```python
from build123d import *

# Parameters (mm, degrees)
SKETCH_W        = 74.53746
SKETCH_H        = 38
PAD_DEPTH       = 2
SKETCH001_W     = 6.85
SKETCH001_H     = 15
PAD001_DEPTH    = 20
SKETCH002_R     = 1.5
POCKET_DEPTH    = 17
SKETCH003_R     = 1.5
PAD002_DEPTH    = 2
SKETCH004_R     = 2.95
PAD003_DEPTH    = 5
SKETCH005_R     = 2.7
SKETCH005_R_2   = 1.5
PAD004_DEPTH    = 2
SKETCH006_W     = 7.7
SKETCH006_H     = 20
SKETCH006_R     = 2.7
PAD005_DEPTH    = 3
SKETCH007_R     = 1.5
PAD006_DEPTH    = 13
SKETCH008_R     = 1.5
PAD007_DEPTH    = 13
FILLET_R        = 3
FILLET001_R     = 5
FILLET002_R     = 1
CHAMFER_SIZE    = 2
CHAMFER001_SIZE = 2


with BuildPart() as body:
    # Sketch → Pad (new body)
    with BuildSketch(Plane.XY):
        Rectangle(SKETCH_W, SKETCH_H)
    extrude(amount=PAD_DEPTH)

    # Sketch001 (on Face6 of Pad) → Pad001 (join)
    with BuildSketch(Plane.XY.offset(2)):
        with Locations((33.84373, -1.3)):
            Rectangle(SKETCH001_W, SKETCH001_H)
        with Locations((-13.60627, -1.3)):
            Rectangle(SKETCH001_W, SKETCH001_H)
    extrude(amount=PAD001_DEPTH)

    # Sketch002 (on Face12 of Pad001) → Pocket (cut)
    with BuildSketch(Plane.XZ.offset(8.8)):
        with Locations((-14.03127, 17)):
            Circle(SKETCH002_R)
        with Locations((-14.03127, 7)):
            Circle(SKETCH002_R)
        with Locations((34.26873, 17)):
            Circle(SKETCH002_R)
        with Locations((34.26873, 7)):
            Circle(SKETCH002_R)
    extrude(amount=-POCKET_DEPTH, mode=Mode.SUBTRACT)

    # Sketch003 (on Face6 of Pocket) → Pad002 (join)
    with BuildSketch(Plane.XZ.offset(19)):
        with BuildLine():
            Line((37.26873, 0), (-37.26873, 0))
            ThreePointArc((-37.26873, 22), (-48.26873, 11), (-37.26873, 0))
            Line((-37.26873, 22), (27.26873, 22))
            ThreePointArc((37.26873, 12), (34.339798, 19.071068), (27.26873, 22))
            Line((37.26873, 12), (37.26873, 0))
        make_face()
        with Locations((-44.73127, 12)):
            Circle(SKETCH003_R, mode=Mode.SUBTRACT)
    extrude(amount=PAD002_DEPTH)

    # Sketch004 (on Face21 of Pad002) → Pad003 (join)
    with BuildSketch(Plane.XZ.offset(21)):
        with Locations((20.26873, 12)):
            Circle(SKETCH004_R)
    extrude(amount=PAD003_DEPTH)

    # Sketch005 (on Face1 of Pad003) → Pad004 (join)
    with BuildSketch(Plane(origin=(0, 19, 0), x_dir=(-1, 0, 0), z_dir=(0, 1, 0))):
        with BuildLine():
            Line((37.26873, 22), (-5.11873, 22))
            ThreePointArc((-5.11873, 22), (-8.654264, 20.535534), (-10.11873, 17))
            Line((-10.11873, 17), (-10.11873, 0))
            Line((-10.11873, 0), (37.26873, 0))
            ThreePointArc((37.26873, 0), (48.26873, 11), (37.26873, 22))
        make_face()
        with Locations((14.03127, 17)):
            Circle(SKETCH005_R, mode=Mode.SUBTRACT)
        with Locations((14.03127, 7)):
            Circle(SKETCH005_R, mode=Mode.SUBTRACT)
        with Locations((44.73127, 12)):
            Circle(SKETCH005_R_2, mode=Mode.SUBTRACT)
    extrude(amount=PAD004_DEPTH)

    # Sketch006 (on Face11 of Pad004) → Pad005 (join)
    with BuildSketch(Plane.XZ.offset(-19)):
        with Locations((-14.03127, 12)):
            Rectangle(SKETCH006_W, SKETCH006_H)
        with Locations((-14.03127, 7)):
            Circle(SKETCH006_R, mode=Mode.SUBTRACT)
        with Locations((-14.03127, 17)):
            Circle(SKETCH006_R, mode=Mode.SUBTRACT)
    extrude(amount=PAD005_DEPTH)

    # Sketch007 (on Face11 of Pad005) → Pad006 (join)
    with BuildSketch(Plane.XZ.offset(-19)):
        with BuildLine():
            ThreePointArc((-41.239359, 12.000001), (-40.426624, 6.534413), (-37.26873, 2))
            Line((-37.26873, 2), (-37.26873, 0))
            ThreePointArc((-48.223181, 11.999999), (-45.392768, 3.583801), (-37.26873, 0))
            ThreePointArc((-41.239359, 12.000001), (-44.731271, 15.491911), (-48.223181, 11.999999))
        make_face()
        with Locations((-44.73127, 12)):
            Circle(SKETCH007_R, mode=Mode.SUBTRACT)
    extrude(amount=PAD006_DEPTH)

    # Sketch008 (on Face20 of Pad006) → Pad007 (join)
    with BuildSketch(Plane(origin=(0, -19, 0), x_dir=(-1, 0, 0), z_dir=(0, 1, 0))):
        with BuildLine():
            Line((37.26873, 2), (37.26873, 0))
            ThreePointArc((37.26873, 0), (45.392768, 3.583802), (48.223181, 12))
            ThreePointArc((48.223181, 12), (44.73127, 15.491911), (41.239359, 12))
            ThreePointArc((37.26873, 2), (40.426624, 6.534412), (41.239359, 12))
        make_face()
        with Locations((44.73127, 12)):
            Circle(SKETCH008_R, mode=Mode.SUBTRACT)
    extrude(amount=PAD007_DEPTH)

    # Fillet
    fillet_edges = [body.edges().sort_by_distance(p)[0] for p in [
        (37.26873, -1.3, 22),
    ]]
    fillet(fillet_edges, radius=FILLET_R)

    # Fillet001
    fillet001_edges = [body.edges().sort_by_distance(p)[0] for p in [
        (37.26873, 19, 1),
    ]]
    fillet(fillet001_edges, radius=FILLET001_R)

    # Fillet002
    fillet002_edges = [body.edges().sort_by_distance(p)[0] for p in [
        (17.31873, -26, 12),
    ]]
    fillet(fillet002_edges, radius=FILLET002_R)

    # Chamfer
    chamfer_edges = [body.edges().sort_by_distance(p)[0] for p in [
        (-10.18127, 19, 12),
    ]]
    chamfer(chamfer_edges, length=CHAMFER_SIZE)

    # Chamfer001
    chamfer001_edges = [body.edges().sort_by_distance(p)[0] for p in [
        (-17.88127, 19, 12),
    ]]
    chamfer(chamfer001_edges, length=CHAMFER001_SIZE)


with BuildPart() as part_mirroring:
    # Part__Mirroring: instance of Body
    add(body.part.mirror(Plane(origin=(0, 0, 0), x_dir=(1, 0, 0), z_dir=(0, 1, 0))))


solid = part_mirroring.part
```
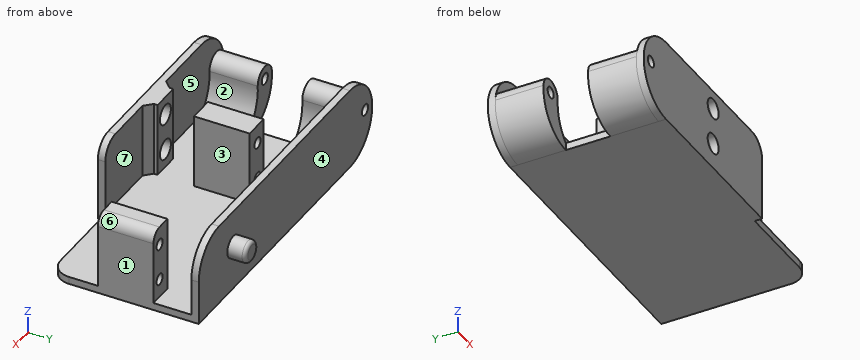
Work out the finished part from the listing and answer in its coordinate system (mm). Face numbers are marked on the shaded views. A direction names the side the tool comes from. Give positions to 0.01 mm unless a question says otherwise; leave off trailing zeros. Loops run counter-clockwise (first coordinate to the right, second up) from the corner with the lowest first, then second, coordinate; pieces in that order, holes last. Notation, with made-up numbers: (21, 68.25) -> (65, 68.25) arc R17 cw to (65, 85.25) -> close; hole circle Ø7 at (-13, 47.5). An arc over 180 degrees is marked (long way). Write item = value, one per line. Start each with the question number.
(1) Find section C-C on z = 7. Give the number of separate pieces and of enclosed holes in the cut face, and give its area (3 significant figures).
(2) Find the intervals of material crossed by probe 1 along Y at (x, z) = (-14, 11.5); probe 2 along Y at (x, z) = (5, 2.25); probe 3 along X at (y, z) = (-2, 15), in increasing order. Write a range as from..to.
(3) The mould has two halves that part along Y. Classify the marked faces 1, 2, 3 and 4: +Y half, -Y half, draft (parallel to the pull), parting line (faces both ways), or undercut.
(4) Which of the six approach directions +Z, -Z, +X, -X, +Y, -Y give full straight-line access (tool end or side, diameter ignored) to the marked faces 5, 6 and 7?
(5) Find section A-A on y = 16.5. Give the vertices of the cut face in (x, z), and give its area (3 significant figures).
(6) Find section B-B on y = -0.5. Give the vertices of the cut face in (x, z), and give its area (3 significant figures).
(7) Find section D-D on x = 16.5. Give the vertices of the cut face in (y, z).
(8) Given pin 1 Ø3.5 at (x, z) = (-44.73, 12) entering from +Y; pin 2 Ø1.5 at (x, y) = (13, 5) entering from +Z; pin 3 Ø5.5 at (x, z) = (33.5, 8) entering from -Y, each flat-ended and moving along its own axis, determine where each tip first touches the part or whether it passes through.
From the geometry:
q1.separate_pieces = 7
q1.enclosed_holes = 0
q1.area = 580 mm^2
q2.probe_1 = -21..-16, -6.2..8.8, 19..21
q2.probe_2 = -21..-19, 19..21
q2.probe_3 = -17.03..-10.18, 30.42..37.27
q3.face_1 = draft
q3.face_2 = undercut
q3.face_3 = undercut
q3.face_4 = +Y half
q4.face_5 = +Z
q4.face_6 = +Z, +X, +Y, -Y
q4.face_7 = +Z, +X
q5.outline = (-48.22, 12) arc R11 ccw to (-37.27, 0) -> (37.27, 0) -> (37.27, 2) -> (-37.27, 2) arc R12.1 cw to (-41.24, 12) arc R3.49 ccw to start; hole circle Ø3 at (-44.73, 12)
q5.area = 238 mm^2
q6.outline = (-37.27, 0) -> (37.27, 0) -> (37.27, 19) arc R3 ccw to (34.27, 22) -> (30.42, 22) -> (30.42, 2) -> (-10.18, 2) -> (-10.18, 22) -> (-17.03, 22) -> (-17.03, 2) -> (-37.27, 2) -> close; hole circle Ø3 at (-14.03, 7); hole circle Ø3 at (-14.03, 17); hole circle Ø3 at (34.27, 7); hole circle Ø3 at (34.27, 17)
q6.area = 393 mm^2
q7.outline = (-19, 0) -> (21, 0) -> (21, 22) -> (19, 22) -> (19, 2) -> (-19, 2) -> close
q8.pin_1 = 21
q8.pin_2 = 2
q8.pin_3 = -6.2
